Drawing for the job (mm, zero at the part's lowest x, y, z). Round coordinates to 2 decimals unless told otherwise and drop trailing zeros. Write each loop counter-clockwise with the first axis right and the second up, starting at its lowest first coordinate (ties: lowest second). Pieces come first, ordered by that corner, then holes.
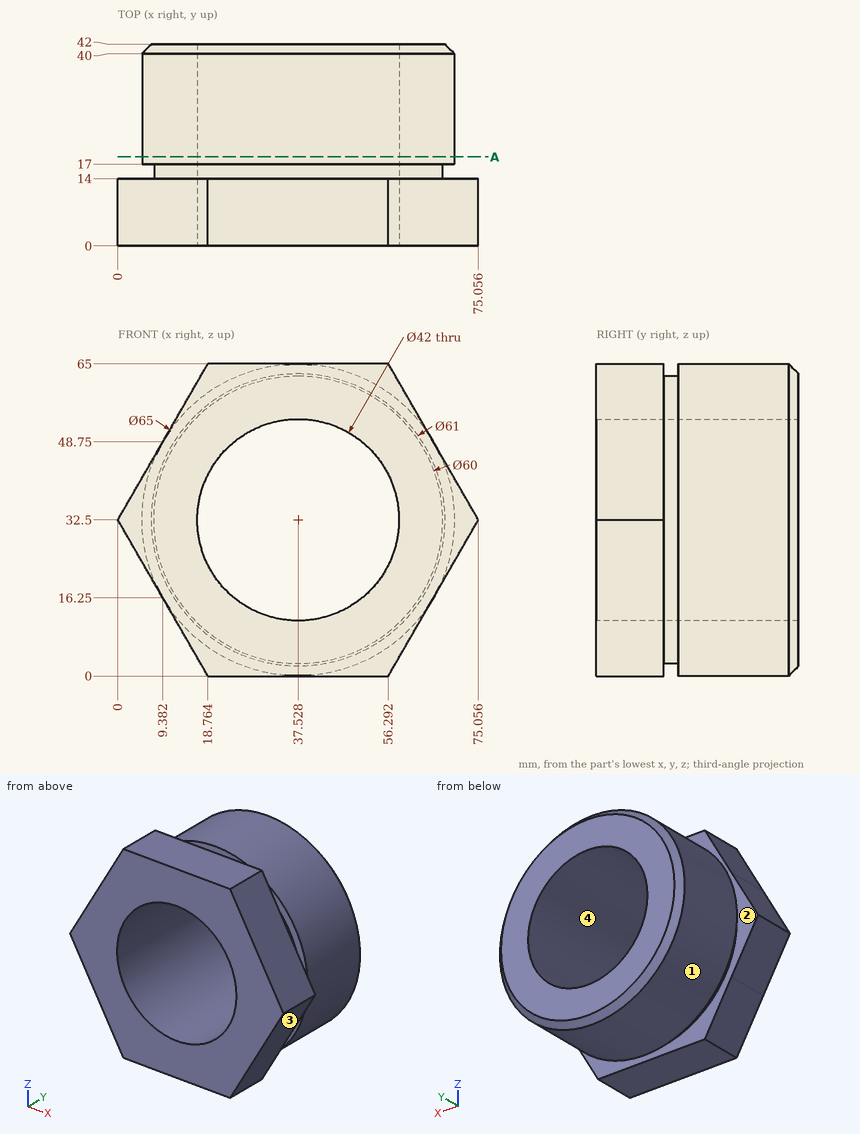
Q1. Drop flat-ended pins along their axis: P1, Ø5, axis at x = 54.5, y = 17, coming from the +Z side; P2, Ø10, axis at x = 62, y = 10, coming from the -Z side (1 decimal); P3, Ø2, axis at x = 13.5, y = 5.5, coming from the +Z side (1 decimal); P4, Ø25, axis at x = 37.53, z = 32.5, coming from the -Y side. Give the stop position or say it passes through.
Q2. Saw through at A-A, the plane y = 18.5. Write the cut outline in (x, z), and give its area (3 significant figures).
Q3. Wall check: line 1 (X direction, y = 33, z = 32); line 2 (X direction, y = 14.5, z = 32.5); line 3 (Z direction, x = 30, y = 18.5) (1 decimal). Give the ranges that are in metal, low to high.
Q4. Two-plate mould, pull along Z, no slides. Class the marked faces 1, 2, 3 and 4: released by +Z, released by -Z, zero draft, split by the parting line, or undercut.
Computed:
1. P1: stops at z = 61.6
1. P2: stops at z = 1.2
1. P3: stops at z = 57.6
1. P4: passes through
2. outline: circle Ø65 at (37.53, 32.5); hole circle Ø42 at (37.53, 32.5)
2. area: 1,930 mm2
3. line 1: x = 5.03 to 16.53, 58.52 to 70.02
3. line 2: x = 7.53 to 16.53, 58.53 to 67.53
3. line 3: z = 0.9 to 12.9, 52.1 to 64.1
4. face 1: split by the parting line
4. face 2: zero draft
4. face 3: released by -Z
4. face 4: undercut
